Source: CAD feature listing. Evaluate the final solid. Frame: model axes, mm. A direction names the side the tool comes from. Coordinates: 2 decimals unless noted, no trailing zeros. Loops run counter-clockwise (first coordinate to the right, second up) from the corner with the lowest first, then second, coordinate; pieces in that order, holes last.
Item 1: Section query C-C, the plane x = -23.5. Return the cut outline in (y, z), then the cut area to 3 significant figures.
Item 2: Line query: probe 1 along Z at (x, y) = (42, 16.5); probe 2 along X at (y, z) = (8, 36); probe 3 along Y at (x, z) = (-49.5, 38). Output: solid intervals per line, ascending.
Item 3: Pin query (flat end, axial travel): pin 1 Ø3 at (x, z) = (31, 21) entering from +Y; pin 2 Ø4 at (x, z) = (-19, 40.5) entering from +Y. Return the tip coordinate at first contact, or that it passes through.
Item 4: Reachability of faces 4 (the flat face through (-10, 6, 35)), 5 (the flat face through (-1, 0, 35)) from +Z, -Z, +X, -X, +Y, -Y: full face, straight path, thin tool, end or side. Return the list, or none.
Item 5: Section query A-A, the plane y = 11.75. Return the cut outline in (x, z).
Item 6: Pull-direction query (X, two-part tool) for faces 1 (the flat face through (-1, 11, 0)), 2 (the flat face through (70, 11, 35)), 3 (the flat face through (-1, 13, 66)); classes: +X half, -X half, draft (parallel to the pull), parting line (faces both ways), or undercut.
```python
from build123d import *

# Parameters (mm, degrees)
SKETCH1_W         = 140
SKETCH1_H         = 70
TRAY_DEPTH        = 22
BASIN_START       = 22
SKETCH2_W         = 132
SKETCH2_H         = 62
BASIN_DEPTH       = 18
GRILLE_RIBS_START = 4
SKETCH3_W         = 4
SKETCH3_H         = 60
GRILLE_RIBS_DEPTH = 2


with BuildPart() as part:
    # Sketch1 → Tray (new body)
    with BuildSketch(Plane(origin=(0, 0, 0), x_dir=(1, 0, 0), z_dir=(0, 1, 0))):
        with Locations((0, -35)):
            Rectangle(SKETCH1_W, SKETCH1_H)
    extrude(amount=TRAY_DEPTH)

    # Sketch2 → Basin (cut)
    with BuildSketch(Plane(origin=(0, 0, 0), x_dir=(1, 0, 0), z_dir=(0, 1, 0)).offset(BASIN_START)):
        with Locations((0, -35)):
            Rectangle(SKETCH2_W, SKETCH2_H)
    extrude(amount=-BASIN_DEPTH, mode=Mode.SUBTRACT)

    # Sketch3 → Grille_Ribs (add)
    with BuildSketch(Plane(origin=(0, 0, 0), x_dir=(1, 0, 0), z_dir=(0, 1, 0)).offset(GRILLE_RIBS_START)):
        with Locations((-50, -35)):
            Rectangle(SKETCH3_W, SKETCH3_H)
        with Locations((-30, -35)):
            Rectangle(SKETCH3_W, SKETCH3_H)
        with Locations((-10, -35)):
            Rectangle(SKETCH3_W, SKETCH3_H)
        with Locations((10, -35)):
            Rectangle(SKETCH3_W, SKETCH3_H)
        with Locations((30, -35)):
            Rectangle(SKETCH3_W, SKETCH3_H)
        with Locations((50, -35)):
            Rectangle(SKETCH3_W, SKETCH3_H)
    extrude(amount=GRILLE_RIBS_DEPTH)


solid = part.part
```
Verdict:
1. outline: (0, 0) - (22, 0) - (22, 4) - (4, 4) - (4, 66) - (22, 66) - (22, 70) - (0, 70) - close
1. area: 424 mm2
2. probe 1: z = 0 to 4, 66 to 70
2. probe 2: x = -70 to -66, 66 to 70
2. probe 3: y = 0 to 6
3. pin 1: stops at y = 6
3. pin 2: stops at y = 4
4. face 4: +Y
4. face 5: +Z, -Z, +X, -X, -Y
5. outline: (-70, 0) - (70, 0) - (70, 70) - (-70, 70) - close; hole (-66, 4) - (66, 4) - (66, 66) - (-66, 66) - close
6. face 1: draft
6. face 2: +X half
6. face 3: undercut
